from build123d import *

# Parameters (mm, degrees)
BOSS_EXTRUDE1_DEPTH = 27
SKETCH2_W           = 40.6
SKETCH2_H           = 30
CUT_EXTRUDE1_DEPTH  = 50.101934789
CUT_EXTRUDE2_DEPTH  = 50.101934789


with BuildPart() as part:
    # Sketch1 → Boss-Extrude1 (new, symmetric)
    with BuildSketch(Plane.XY):
        Polygon((-29, 0), (0, 0), (0, 29), (1, 29), (1, -1), (-29, -1), align=None)
    extrude(amount=BOSS_EXTRUDE1_DEPTH, both=True)

    # Sketch2 → Cut-Extrude1 (cut, through all)
    with BuildSketch(Plane.ZY):
        with BuildLine():
            Line((-24.5, 17), (-27, 17))
            Line((-27, 17), (-27, 13))
            Line((-27, 13), (-24.5, 13))
            ThreePointArc((-24.5, 13), (-22.5, 15), (-24.5, 17))
        make_face()
        with Locations((0, 15)):
            Rectangle(SKETCH2_W, SKETCH2_H)
        with BuildLine():
            Line((-24.5, 3), (-27, 3))
            Line((-27, 3), (-27, 7))
            Line((-27, 7), (-24.5, 7))
            ThreePointArc((-24.5, 7), (-22.5, 5), (-24.5, 3))
        make_face()
        with BuildLine():
            Line((24.5, 7), (27, 7))
            Line((27, 7), (27, 3))
            Line((27, 3), (24.5, 3))
            ThreePointArc((24.5, 3), (22.5, 5), (24.5, 7))
        make_face()
        with BuildLine():
            Line((24.5, 13), (27, 13))
            Line((27, 13), (27, 17))
            Line((27, 17), (24.5, 17))
            ThreePointArc((24.5, 17), (22.5, 15), (24.5, 13))
        make_face()
    extrude(amount=-CUT_EXTRUDE1_DEPTH, mode=Mode.SUBTRACT)

    # Sketch3 → Cut-Extrude2 (cut, through all)
    with BuildSketch(Plane(origin=(0, 0, 0), x_dir=(1, 0, 0), z_dir=(0, 1, 0))):
        with BuildLine():
            ThreePointArc((-16, 23), (-14, 21), (-12, 23))
            ThreePointArc((-12, 23), (-14, 25), (-16, 23))
        make_face()
        with BuildLine():
            ThreePointArc((-12, -23), (-14, -21), (-16, -23))
            ThreePointArc((-16, -23), (-14, -25), (-12, -23))
        make_face()
    extrude(amount=-CUT_EXTRUDE2_DEPTH, mode=Mode.SUBTRACT)


solid = part.part
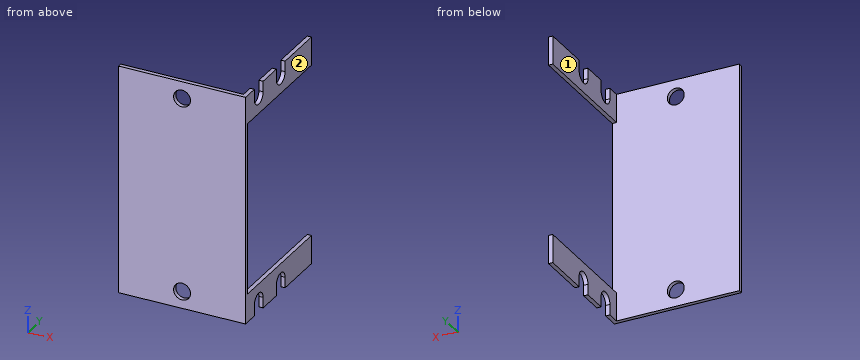
Verification items for the finished model (mm, model axes). Face numbers are marked on the shaded views. A direction names the side the tool comes from. Give positions to 0.01 mm unless a question says otherwise; leave off trailing zeros. Write each loop counter-clockwise with the first axis right and the second up, starting at its lowest first coordinate (ties: lowest second). Pieces come first, ordered by that corner, then holes. Notation, with made-up numbers: M 43.25,83 L 71.25,83 A13 cw 71.25,94 Z; hole C 3,58 d7. An arc over 180 degrees is marked long. Put each result on its own line as item: value. Start each with the question number.
1. Section check D-D (z = 8). Record the cut outline in (x, y), and give its area (3 significant figures).
2. Scan lines: line 1 along Z through (x, y) = (-14, -0.45); line 2 along Y through (x, z) = (-13.25, -10.5); line 3 along X through (y, z) = (7.5, 24.5). Record each from-to range of solid material in increasing order. Write a range as [from, to].
3. Go/stop test with flat-tipped pins: pin 1 Ø0.5 at (x, y) = (0.5, 13.5) entering from +Z; pin 2 Ø3.5 at (y, z) = (10, 22.5) entering from -X; pin 3 Ø4 at (x, z) = (-11.5, -0.5) entering from +Y. Record where each tip stops, or that it passes through.
4. Section check B-B (x = -14). Record the cut outline in (y, z), and give its area (3 significant figures).
5. Set-up check for the marked faces 1 and 2: record each of +Z, -Z, +X, -X, +Y, -Y from which the full face is reachable in a straight line by a thin tool's end or side.
6. Section check A-A (y = 5). Record the cut outline in (x, z).
7. Section check C-C (y = 1.75). Record the cut outline in (x, z), and give its area (3 significant figures).
Answer list:
1. outline: M -29,-1 L 1,-1 L 1,0 L -29,0 Z
1. area: 30.0 mm2
2. line 1: [-27, -25], [-21, 21], [25, 27]
2. line 2: [-1, 0]
2. line 3: [0, 1]
3. pin 1: z = 23.53
3. pin 2: x = 0
3. pin 3: y = 0
4. outline: M -1,-27 L 0,-27 L 0,-25 L -1,-25 Z; M -1,-21 L 0,-21 L 0,21 L -1,21 Z; M -1,25 L 0,25 L 0,27 L -1,27 Z
4. area: 46.0 mm2
5. face 1: +Z, -Z, -X, +Y
5. face 2: +Z, -Z, +X, +Y, -Y
6. outline: M 0,-22.5 L 1,-22.5 L 1,-20.3 L 0,-20.3 Z; M 0,20.3 L 1,20.3 L 1,22.5 L 0,22.5 Z
7. outline: M 0,-27 L 1,-27 L 1,-20.3 L 0,-20.3 Z; M 0,20.3 L 1,20.3 L 1,27 L 0,27 Z
7. area: 13.4 mm2
